Geometry check sheet. Reference: the model listing, model coordinates, mm. A direction names the side the tool comes from. Round coordinates to 2 decimals unless told otherwise and drop trailing zeros. Loops run counter-clockwise (first coordinate to the right, second up) from the corner with the lowest first, then second, coordinate; pieces in that order, holes last.
```python
from build123d import *

# Parameters (mm, degrees)
SKETCH1_W           = 8
SKETCH1_H           = 28
BOSS_EXTRUDE2_DEPTH = 60
CUT_EXTRUDE2_DEPTH  = 65.353734654
SKETCH6_R           = 1.5
CUT_EXTRUDE3_DEPTH  = 25
SKETCH7_W           = 5.7
SKETCH7_H           = 3
CUT_EXTRUDE4_DEPTH  = 65.353734654
SKETCH8_R           = 1.5
CUT_EXTRUDE5_DEPTH  = 25


with BuildPart() as part:
    # Sketch1 → Boss-Extrude2 (new body)
    with BuildSketch(Plane(origin=(0, 0, 0), x_dir=(1, 0, 0), z_dir=(0, 1, 0))):
        with Locations((6, 7.849557522)):
            Rectangle(SKETCH1_W, SKETCH1_H)
    extrude(amount=BOSS_EXTRUDE2_DEPTH)

    # Sketch5 → Cut-Extrude2 (cut, through all)
    with BuildSketch(Plane(origin=(10, 0, 0), x_dir=(0, 0, -1), z_dir=(1, 0, 0))):
        with BuildLine():
            Line((-0.087696411, 0), (15.786811455, 0))
            ThreePointArc((15.786811455, 0), (7.849557522, 7), (-0.087696411, 0))
        make_face()
    extrude(amount=-CUT_EXTRUDE2_DEPTH, mode=Mode.SUBTRACT)

    # Sketch6 → Cut-Extrude3 (cut)
    with BuildSketch(Plane.XZ):
        with Locations(Location((6, -18.349557522, 0), (0, 0, 270))):
            Circle(SKETCH6_R)
        with Locations(Location((6, 2.650442478, 0), (0, 0, 270))):
            Circle(SKETCH6_R)
    extrude(amount=-CUT_EXTRUDE3_DEPTH, mode=Mode.SUBTRACT)

    # Sketch7 → Cut-Extrude4 (cut, through all)
    with BuildSketch(Plane.ZY.offset(-2)):
        with Locations((-15.999557522, 53.5)):
            Rectangle(SKETCH7_W, SKETCH7_H)
        with Locations((0.300442478, 53.5)):
            Rectangle(SKETCH7_W, SKETCH7_H)
    extrude(amount=-CUT_EXTRUDE4_DEPTH, mode=Mode.SUBTRACT)

    # Sketch8 → Cut-Extrude5 (cut)
    with BuildSketch(Plane(origin=(0, 60, 0), x_dir=(1, 0, 0), z_dir=(0, 1, 0))):
        with Locations(Location((6, 15.999557522, 0), (0, 0, 270))):
            Circle(SKETCH8_R)
        with Locations(Location((6, -0.300442478, 0), (0, 0, 270))):
            Circle(SKETCH8_R)
    extrude(amount=-CUT_EXTRUDE5_DEPTH, mode=Mode.SUBTRACT)


solid = part.part
```
1) Scan lines: line 1 along Z through (x, y) = (7, 44.5); line 2 along Z through (x, y) = (5.75, 6); line 3 along Z through (x, y) = (5, 24). Record each from-to range of solid material in increasing order.
Report:
line 1: z = -21.85 to -17.12, -14.88 to -0.82, 1.42 to 6.15
line 2: z = -21.85 to -19.83, -16.87 to -11.72, -3.98 to 1.17, 4.13 to 6.15
line 3: z = -21.85 to -19.47, -17.23 to 1.53, 3.77 to 6.15
2) Gauge pin test, flat ends, axial feed: pin 1 (2.5 mm diameter, centred on x = 6, z = 0.3, fed in from +Y); pin 2 (2.5 mm diameter, centred on x = 6, z = -17.5, fed in from -Y). Record the tip position at first contact, or that the pin passes through.
Report:
pin 1: stops at y = 35
pin 2: stops at y = 0
3) Mould release check, pull along X, two halves, no side actions. Record for faces 5 (the face through (6, 35, -16)), 6 (the face through (10, 30, -8)), 7 (the face through (6, 60, -8)): +X half, -X half, draft (parallel to the pull), parting line (faces both ways), or undercut.
Report:
face 5: undercut
face 6: +X half
face 7: draft
4) Sectioned sample at A-A, the plane z = -15.25. Record the cut outline in (x, y), then the cut area to 3 significant figures.
Report:
outline: (2, 2.04) - (10, 2.04) - (10, 52) - (7.3, 52) - (7.3, 35) - (4.7, 35) - (4.7, 52) - (2, 52) - close; (2, 55) - (4.7, 55) - (4.7, 60) - (2, 60) - close; (7.3, 55) - (10, 55) - (10, 60) - (7.3, 60) - close
area: 383 mm2
5) Sectioned sample at B-B, the plane y = 23. Record the cut outline in (x, z).
Report:
outline: (2, -21.85) - (10, -21.85) - (10, 6.15) - (2, 6.15) - close; hole circle Ø3 at (6, -18.35); hole circle Ø3 at (6, 2.65)
6) Access from +Z, -Z, +X, -X, +Y, -Y to the whole of each face (thin tool, end or side, straight path). Record for faces 1 (the face through (6, 53, -18.85)), 2 (the face through (5.43, 57.54, -14.61)), 3 (the face through (6, 25, -18)), 4 (the face through (5.9, 0, 4.4)).
Report:
face 1: +X, -X
face 2: +Y
face 3: -Y
face 4: +Z, -Z, +X, -X, -Y
7) Sectioned sample at C-C, the plane z = -11.5. Record the cut outline in (x, y), then the cut area to 3 significant figures.
Report:
outline: (2, 6.12) - (10, 6.12) - (10, 60) - (2, 60) - close
area: 431 mm2
